Can you work these out from the model? Positions are in its coordinate system, mm. A direction names the side the tool comes from. Coordinates: 2 decimals unless noted, no trailing zeros. Order: outer loops, then holes, each group sorted by start corner. A loop starts at its lowest first (then second) coordinate and runs counter-clockwise, first axis right, second up. Notation, with made-up numbers: (17.25, -35.5) -> (35.25, -35.5) arc R21 cw to (35.25, -31.5) -> close; hole circle Ø5 at (-32.75, 6.5). An arc over 180 degrees is marked (long way). Answer as CSV lines item,"result".
from build123d import *

# Parameters (mm, degrees)
F0_R     = 25
F0_R_2   = 6
F1_DEPTH = 4
F0_R_3   = 4
F2_DEPTH = 8
F5_DEPTH = 25
F6_R     = 6
F6_R_2   = 1.25
F7_DEPTH = 4


with BuildPart() as f1:
    # F0 (on Top) → F1 (new body)
    with BuildSketch(Plane.XY):
        Circle(F0_R)
        Circle(F0_R_2, mode=Mode.SUBTRACT)
    extrude(amount=F1_DEPTH)

    # F0 (on Top) → F2 (join)
    with BuildSketch(Plane.XY):
        Circle(F0_R_2)
        Circle(F0_R_3, mode=Mode.SUBTRACT)
    extrude(amount=F2_DEPTH)

    # F4 (on face) → F5 (cut)
    with BuildSketch(Plane.XY.offset(4)):
        with BuildLine():
            ThreePointArc((8.561512, 17.523658), (-0.015533, 19.478312), (-8.581679, 17.47643))
            Line((-8.581679, 17.47643), (-6.362037, 13.037147))
            ThreePointArc((-6.362037, 13.037147), (0.01353, 14.496219), (6.389097, 13.037147))
            Line((6.389097, 13.037147), (8.561512, 17.523658))
        make_face()
    extrude(amount=-F5_DEPTH, mode=Mode.SUBTRACT)

    # F6 (on face) → F7 (join)
    with BuildSketch(Plane.XY.offset(8)):
        Circle(F6_R)
        Circle(F6_R_2, mode=Mode.SUBTRACT)
    extrude(amount=F7_DEPTH)


solid = f1.part
Q1. Which directions (+Z, -Z, +X, -X, +Y, -Y) give clear straight access to the entire face, cutting with the end or side of a thin tool? Please do faces 1 (the cylindrical face through (-0.867, -3.905, 3.944)), 2 (the flat face through (0, -5, 0)), 3 (the flat face through (5, -5, 4)), 4 (the flat face through (-7.49, 15.29, 2.03)).
Solution:
face 1,"-Z"
face 2,"-Z, +X, -X, +Y, -Y"
face 3,"+Z"
face 4,"+Z, -Z"
Q2. If I drill on line 1 (Y direction, x = 0, z = 3.5); line 2 (Y direction, x = 0, z = 9.35); line 3 (Y direction, x = 1.5, z = 2), over which ranges is the centre line in solid material (lowest first)?
Solution:
line 1,"-25 to -4, 4 to 14.5, 19.48 to 25"
line 2,"-6 to -1.25, 1.25 to 6"
line 3,"-24.95 to -3.71, 3.71 to 14.42, 19.42 to 24.95"
Q3. Imagine slicing it at D-D (z = 10.25). List the corners of the cut face in (x, y) for me.
Solution:
outline,"circle Ø12 at (0, 0); hole circle Ø2.5 at (0, 0)"
Q4. We'd pull the mould along Y, two halves only. Please class faces 5 (the flat face through (-0.1, 1.4, 12)), 6 (the cylindrical face through (-6, 0, 8)), 7 (the flat face through (-1, -1, 8)): pulls with the +Y half, pulls with the -Y half, needs draft (parallel to the pull), parting line crosses it, or undercut.
Solution:
face 5,"needs draft"
face 6,"parting line crosses it"
face 7,"undercut"
Q5. Imagine slicing it at A-A (y = 0). List the corners of the cut face in (x, z) for me, and give its area (3 significant figures).
Solution:
outline,"(-25, 0) -> (-4, 0) -> (-4, 8) -> (-1.25, 8) -> (-1.25, 12) -> (-6, 12) -> (-6, 4) -> (-25, 4) -> close; (1.25, 8) -> (4, 8) -> (4, 0) -> (25, 0) -> (25, 4) -> (6, 4) -> (6, 12) -> (1.25, 12) -> close"
area,"222 mm2"
Q6. Imagine slicing it at C-C (z = 1.5). List the corners of the cut face in (x, y) for me.
Solution:
outline,"circle Ø50 at (0, 0); hole (-8.58, 17.48) -> (-6.36, 13.04) arc R14.66 cw to (6.39, 13.04) -> (8.56, 17.52) arc R19.56 ccw to start; hole circle Ø8 at (0, 0)"
Q7. Imagine slicing it at B-B (x = 2). List the corners of the cut face in (y, z) for me, and give its area (3 significant figures).
Solution:
outline,"(-24.92, 0) -> (-3.46, 0) -> (-3.46, 8) -> (3.46, 8) -> (3.46, 0) -> (14.36, 0) -> (14.36, 4) -> (5.66, 4) -> (5.66, 12) -> (-5.66, 12) -> (-5.66, 4) -> (-24.92, 4) -> close; (19.38, 0) -> (24.92, 0) -> (24.92, 4) -> (19.38, 4) -> close"
area,"214 mm2"
Q8. For P1, Ø4, axis at x = 0.5, y = -0.5, coming from the -Z side; P2, Ø2, axis at x = 0, y = 0, coming from the +Z side; P3, Ø5, axis at x = -2.5, z = 4.5, coming from the -Y side; P4, Ø10, axis at x = -10.5, y = 17, coming from the +Z side, each with a flat end and sliding along its axis, tell me the tip position at first contact or that it passes through.
Solution:
P1,"z = 8"
P2,"through"
P3,"y = -25"
P4,"z = 4"
